Build history of the part. All positions in model axes, mm. Face numbers are marked on the shaded views. A direction names the side the tool comes from. Give positions to 0.01 mm unless a question says otherwise; leave off trailing zeros. Loops run counter-clockwise (first coordinate to the right, second up) from the corner with the lowest first, then second, coordinate; pieces in that order, holes last. Notation, with made-up numbers: M 85,2 L 107,2 A18 ccw 107,15 Z; hole C 62,9.5 d1. An arc over 180 degrees is marked long. Answer as a JSON object with one key per item and string values. Group by question number.
1. Slice it at B-B (x = 14.5). List the corners of the cut face in (y, z), then the cut area to 3 significant figures.
2. Slice it at C-C (z = -10). List the corners of the cut face in (x, y), then the cut area to 4 significant figures.
3. Slice it at D-D (z = -31). List the corners of the cut face in (x, y), then the cut area to 3 significant figures.
4. 3-axis set-ups, long thin cutter, end or side, ignore diameter. For the marked faces 1 and 2: which of +Z, -Z, +X, -X, +Y, -Y reach the whole face in a straight line?
5. Drop flat-ended pins along their axis: pin 1 Ø1.6 at (x, y) = (23.26, -4.24) entering from -Z; pin 2 Ø4 at (x, z) = (4, -26) entering from -Y. Give the stop position or say it passes through.
6. Slice it at A-A (y = -6). List the corners of the cut face in (x, z), then the cut area to 3 significant figures.
7. Drill centre lines: line 1 along Y through (x, z) = (-27.5, -35.5); line 2 along Z through (x, y) = (12, -5.5); line 3 along Y through (x, z) = (27, 1). Where is each one in solid material? Low to high. Write a range as [from, to].
8. Mould opens along Z. For the marked faces 3, 4 and 5 say: released by +Z, released by -Z, zero draft, split by the parting line, or undercut.
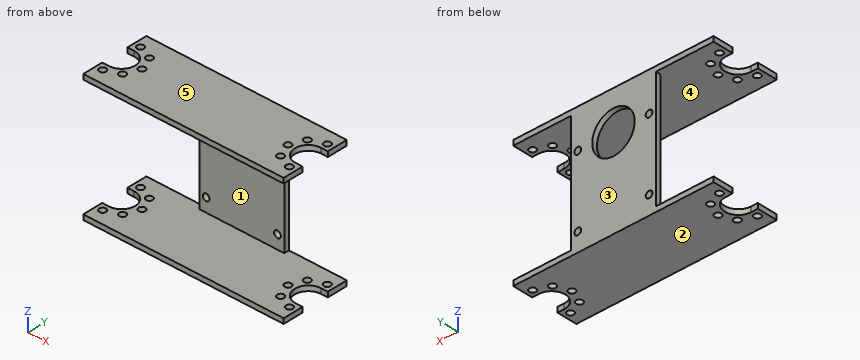
from build123d import *

# Parameters (mm, degrees)
F0_R     = 1
F1_DEPTH = 1.5
F2_W     = 25
F2_H     = 1.5
F3_DEPTH = 17.5
F6_R     = 1
F6_R_2   = 6.25
F7_DEPTH = 1.5


with BuildPart() as f1:
    # F0 (on Top) → F1 (new body)
    with BuildSketch(Plane.XY):
        with BuildLine():
            Line((-29.5, -10), (29.5, -10))
            Line((29.5, -10), (29.5, -4))
            Line((29.5, -4), (27.5, -4))
            ThreePointArc((27.5, -4), (23.5, 0), (27.5, 4))
            Line((27.5, 4), (29.5, 4))
            Line((29.5, 4), (29.5, 10))
            Line((29.5, 10), (-29.5, 10))
            Line((-29.5, 10), (-29.5, 4))
            Line((-29.5, 4), (-27.5, 4))
            ThreePointArc((-27.5, 4), (-23.5, 0), (-27.5, -4))
            Line((-27.5, -4), (-29.5, -4))
            Line((-29.5, -4), (-29.5, -10))
        make_face()
        with Locations((-27.5, -6)):
            Circle(F0_R, mode=Mode.SUBTRACT)
        with Locations((-23.257359, -4.242641)):
            Circle(F0_R, mode=Mode.SUBTRACT)
        with Locations((27.5, -6)):
            Circle(F0_R, mode=Mode.SUBTRACT)
        with Locations((23.257359, -4.242641)):
            Circle(F0_R, mode=Mode.SUBTRACT)
        with Locations((-21.5, 0)):
            Circle(F0_R, mode=Mode.SUBTRACT)
        with Locations((-23.257359, 4.242641)):
            Circle(F0_R, mode=Mode.SUBTRACT)
        with Locations((-27.5, 6)):
            Circle(F0_R, mode=Mode.SUBTRACT)
        with Locations((21.5, 0)):
            Circle(F0_R, mode=Mode.SUBTRACT)
        with Locations((23.257359, 4.242641)):
            Circle(F0_R, mode=Mode.SUBTRACT)
        with Locations((27.5, 6)):
            Circle(F0_R, mode=Mode.SUBTRACT)
    extrude(amount=F1_DEPTH)

    # F2 (on face) → F3 (join)
    with BuildSketch(Plane(origin=(0, 0, 0), x_dir=(1, 0, 0), z_dir=(0, 0, -1))):
        with Locations((0, -9.25)):
            Rectangle(F2_W, F2_H)
    extrude(amount=F3_DEPTH)

    # F5: F1 across plane


with BuildPart() as f1_1:
    add(f1.part)
    add(f1.part.mirror(Plane.XY.offset(-17.5)))

    # F6 (on face) → F7 (cut, through all)
    with BuildSketch(Plane(origin=(0, 10, 0), x_dir=(-1, 0, 0), z_dir=(0, 1, 0))):
        with Locations((10.5, -10)):
            Circle(F6_R)
        with Locations((10.5, -31)):
            Circle(F6_R)
        with Locations((0, -10)):
            Circle(F6_R_2)
        with Locations((-10.5, -10)):
            Circle(F6_R)
        with Locations((-10.5, -31)):
            Circle(F6_R)
    extrude(amount=-F7_DEPTH, mode=Mode.SUBTRACT)


solid = f1_1.part
Established:
{
 "1": {"outline": "M -10,-36.5 L 10,-36.5 L 10,-35 L -10,-35 Z; M -10,0 L 10,0 L 10,1.5 L -10,1.5 Z", "area": "60.0 mm^2"},
 "2": {"outline": "M -12.5,8.5 L -11.5,8.5 L -11.5,10 L -12.5,10 Z; M -9.5,8.5 L -6.25,8.5 L -6.25,10 L -9.5,10 Z; M 6.25,8.5 L 9.5,8.5 L 9.5,10 L 6.25,10 Z; M 11.5,8.5 L 12.5,8.5 L 12.5,10 L 11.5,10 Z", "area": "12.75 mm^2"},
 "3": {"outline": "M -12.5,8.5 L -11.5,8.5 L -11.5,10 L -12.5,10 Z; M -9.5,8.5 L 9.5,8.5 L 9.5,10 L -9.5,10 Z; M 11.5,8.5 L 12.5,8.5 L 12.5,10 L 11.5,10 Z", "area": "31.5 mm^2"},
 "4": {"face 1": "+X, -X, -Y", "face 2": "-Z, +X, -X, +Y, -Y"},
 "5": {"pin 1": "passes through", "pin 2": "stops at y = 8.5"},
 "6": {"outline": "M -29.5,-36.5 L -28.5,-36.5 L -28.5,-35 L -29.5,-35 Z; M -29.5,0 L -28.5,0 L -28.5,1.5 L -29.5,1.5 Z; M -26.5,-36.5 L 26.5,-36.5 L 26.5,-35 L -26.5,-35 Z; M -26.5,0 L 26.5,0 L 26.5,1.5 L -26.5,1.5 Z; M 28.5,-36.5 L 29.5,-36.5 L 29.5,-35 L 28.5,-35 Z; M 28.5,0 L 29.5,0 L 29.5,1.5 L 28.5,1.5 Z", "area": "165 mm^2"},
 "7": {"line 1": "y = [-10, -7], [-5, -4], [4, 5], [7, 10]", "line 2": "z = [-36.5, -35], [0, 1.5]", "line 3": "y = [-10, -6.87], [-5.13, -3.97], [3.97, 5.13], [6.87, 10]"},
 "8": {"face 3": "zero draft", "face 4": "undercut", "face 5": "released by +Z"}
}
